The listing builds one solid part. Answer for the finished solid, in the listing's coordinates (mm). A direction names the side the tool comes from. Give positions to 0.01 mm unless a question says otherwise; leave off trailing zeros. Loops run counter-clockwise (first coordinate to the right, second up) from the corner with the lowest first, then second, coordinate; pieces in that order, holes last. Notation, with made-up numbers: M 42,63.5 L 64,63.5 A24 ccw 64,86.5 Z; hole C 0.25,59 d11. An arc over 180 degrees is marked long. One line per item, written item: value. Start each with the question number.
Q1. For faces 1 (the flat face through (30.806, -16, -13)), 2 (the flat face through (13, 8.36, 15)), 3 (the flat face through (29, -12.508, -24)), 4 (the flat face through (12, 11.36, 15)), determine the directions among +Z, -Z, +X, -X, +Y, -Y from which every point of the face is accessible in a straight line to the end or side of a thin tool.
Q2. A cutting plane is placed at C-C, the plane y = -3.5. Determine the outline of the cut face in (x, z), and give its area (3 significant figures).
Q3. A cutting plane is placed at D-D, the plane z = 22.5. Determine the outline of the cut face in (x, y), and give its area (3 significant figures).
Q4. A cutting plane is placed at A-A, the plane z = 8.5. Determine the outline of the cut face in (x, y).
Q5. Consider L1, parallel to Z at x = -10, y = 6; L2, parallel to X at y = -31, z = -17; L3, parallel to Y at x = 29, z = -21. Determine where each line is inside the solid, lowest interval first.
Q6. The mould has two halves that part along X. Classify faces 5 (the cylindrical face through (16.997, 9.839, 7.496)), 6 (the flat face through (27.806, -16, -13)), 7 (the cylindrical face through (32.327, 52.509, 21.277)): +X half, -X half, draft (parallel to the pull), parting line (faces both ways), or undercut.
Q7. A cutting plane is placed at B-B, the plane x = -3. Determine the outline of the cut face in (y, z), and give its area (3 significant figures).
Q8. Flat-ended cylindrical pins translate along their axes: pin 1 (12 mm diameter, centred on y = 30, z = 10.5, fed in from -X); pin 2 (14.5 mm diameter, centred on x = 1.5, z = -2, fed in from +Y); pin 3 (23 mm diameter, centred on x = 14.5, y = -22, fed in from -Z); pin 4 (2 mm diameter, centred on x = -12.69, z = 8.5, fed in from -Y). Find the tip coordinate at first contact, or state that the pin passes through.
from build123d import *

# Parameters (mm, degrees)
SKETCH_1_W          = 42
SKETCH_1_H          = 53
EXTRUDE_1_DEPTH     = 3
SKETCH_2_W          = 42
SKETCH_2_H          = 3
EXTRUDE_2_DEPTH     = 42
SKETCH_3_R          = 12
SKETCH_3_R_2        = 1.65
CUT_EXTRUDE_1_DEPTH = 4
EXTRUDE_3_DEPTH     = 10
SKETCH_5_W          = 3
SKETCH_5_H          = 45
EXTRUDE_4_DEPTH     = 53.5
SKETCH_6_R          = 2.65
CUT_EXTRUDE_2_DEPTH = 20
SKETCH_7_W          = 3
SKETCH_7_H          = 53
EXTRUDE_5_DEPTH     = 33.96
CUT_EXTRUDE_4_DEPTH = 33.96


with BuildPart() as part:
    # 草图1 → 凸台-拉伸1 (new body)
    with BuildSketch(Plane.XY):
        with Locations((2.806034483, -15.140086207)):
            Rectangle(SKETCH_1_W, SKETCH_1_H)
    extrude(amount=EXTRUDE_1_DEPTH)

    # 草图2 → 凸台-拉伸2 (add)
    with BuildSketch(Plane.XY.offset(3)):
        with Locations((2.806034483, 9.859913793)):
            Rectangle(SKETCH_2_W, SKETCH_2_H)
    extrude(amount=EXTRUDE_2_DEPTH)

    # 草图3 → 切除-拉伸1 (cut, through all)
    with BuildSketch(Plane.XZ.offset(-8.359913793)):
        with Locations((2.806034483, 24)):
            Circle(SKETCH_3_R)
        with Locations((18.306034483, 39.5)):
            Circle(SKETCH_3_R_2)
        with Locations((18.306034483, 8.5)):
            Circle(SKETCH_3_R_2)
        with Locations((-12.693965517, 8.5)):
            Circle(SKETCH_3_R_2)
        with Locations((-12.693965517, 39.5)):
            Circle(SKETCH_3_R_2)
    extrude(amount=-CUT_EXTRUDE_1_DEPTH, mode=Mode.SUBTRACT)

    # 草图4 → 凸台-拉伸3 (add)
    with BuildSketch(Plane(origin=(23.806034483, 0, 0), x_dir=(0, 0, -1), z_dir=(1, 0, 0))):
        Polygon((-45, 8.359913793), (-3, 8.359913793), (-3, -41.640086207), (0, -41.640086207), (0, 8.359913793), (0, 11.359913793), (-45, 11.359913793), align=None)
    extrude(amount=EXTRUDE_3_DEPTH)

    # 草图5 → 凸台-拉伸4 (add)
    with BuildSketch(Plane(origin=(0, 11.359913793, 0), x_dir=(1, 0, 0), z_dir=(0, 1, 0))):
        with Locations((32.306034483, -22.5)):
            Rectangle(SKETCH_5_W, SKETCH_5_H)
    extrude(amount=EXTRUDE_4_DEPTH)

    # 草图6 → 切除-拉伸2 (cut)
    with BuildSketch(Plane(origin=(33.806034483, 0, 0), x_dir=(0, 0, -1), z_dir=(1, 0, 0))):
        with Locations((-22.5, 54.859913793)):
            Circle(SKETCH_6_R)
    extrude(amount=-CUT_EXTRUDE_2_DEPTH, mode=Mode.SUBTRACT)

    # 草图7 → 凸台-拉伸5 (add)
    with BuildSketch(Plane(origin=(0, 0, 0), x_dir=(-1, 0, 0), z_dir=(0, 0, -1))):
        with Locations((-29.306034483, -15.140086207)):
            Rectangle(SKETCH_7_W, SKETCH_7_H)
    extrude(amount=EXTRUDE_5_DEPTH)

    # 草图10 → 切除-拉伸4 (cut)
    with BuildSketch(Plane(origin=(30.806034483, 0, 0), x_dir=(0, 0, -1), z_dir=(1, 0, 0))):
        with BuildLine():
            Line((28.96, -17.807711285), (19.224876223, -17.807711285))
            ThreePointArc((19.224876223, -17.807711285), (16.574876223, -15.157711285), (19.224876223, -12.507711285))
            Line((19.224876223, -12.507711285), (28.96, -12.507711285))
            ThreePointArc((28.96, -12.507711285), (31.61, -15.157711285), (28.96, -17.807711285))
        make_face()
    extrude(amount=-CUT_EXTRUDE_4_DEPTH, mode=Mode.SUBTRACT)


solid = part.part
Answer block:
1. face 1: -Z, +X, +Y, -Y
1. face 2: +Z, +X, -X, -Y
1. face 3: +X, -X
1. face 4: +Z, -Z, -X, +Y
2. outline: M -18.19,0 L 27.81,0 L 27.81,-33.96 L 30.81,-33.96 L 30.81,0 L 33.81,0 L 33.81,3 L -18.19,3 Z
2. area: 258 mm^2
3. outline: M -18.19,8.36 L -9.1,8.36 L -9.1,11.36 L -18.19,11.36 Z; M 14.71,8.36 L 33.81,8.36 L 33.81,52.21 L 30.81,52.21 L 30.81,11.36 L 14.71,11.36 Z; M 30.81,57.51 L 33.81,57.51 L 33.81,64.86 L 30.81,64.86 Z
3. area: 229 mm^2
4. outline: M -18.19,8.36 L -14.34,8.36 L -14.34,11.36 L -18.19,11.36 Z; M -11.04,8.36 L 16.66,8.36 L 16.66,11.36 L -11.04,11.36 Z; M 19.96,8.36 L 33.81,8.36 L 33.81,64.86 L 30.81,64.86 L 30.81,11.36 L 19.96,11.36 Z
5. L1: 0 to 3
5. L2: 27.81 to 30.81
5. L3: -41.64 to -17.81, -12.51 to 11.36
6. face 5: undercut
6. face 6: -X half
6. face 7: draft
7. outline: M -41.64,0 L 11.36,0 L 11.36,13.5 L 8.36,13.5 L 8.36,3 L -41.64,3 Z; M 8.36,34.5 L 11.36,34.5 L 11.36,45 L 8.36,45 Z
7. area: 222 mm^2
8. pin 1: x = 30.81
8. pin 2: y = 11.36
8. pin 3: z = 0
8. pin 4: through
